```python
from build123d import *

# Parameters (mm, degrees)
BOX015_W                  = 3
BOX015_H                  = 2.5
BOX015_DEPTH              = 1.5
BOX014_W                  = 3
BOX014_H                  = 2.5
BOX014_DEPTH              = 1.5
CYLINDER009_R             = 1.2
CYLINDER009_DEPTH         = 1.54
CYLINDER010_R             = 1.2
CYLINDER010_DEPTH         = 1.54
CYLINDER011_R             = 4.5
CYLINDER011_DEPTH         = 1.54
CYLINDER012_R             = 4.5
CYLINDER012_DEPTH         = 1.54
BOX013_W                  = 18
BOX013_H                  = 16
BOX013_DEPTH              = 1.54
BOX016_W                  = 16.5
BOX016_H                  = 10
BOX016_DEPTH              = 1.54
FUSION014_ROLL_ANGLE      = 180
FUSION014_PLACEMENT_ANGLE = 90.000069


with BuildPart() as cubo015:
    # Box015 → Box015 (new body)
    with BuildSketch(Plane(origin=(12.5, 21.5, 1.54), x_dir=(1, 0, 0), z_dir=(0, 0, 1))):
        with Locations((1.5, 1.25)):
            Rectangle(BOX015_W, BOX015_H)
    extrude(amount=BOX015_DEPTH)


with BuildPart() as cubo014:
    # Box014 → Box014 (new body)
    with BuildSketch(Plane(origin=(3, 21.5, 1.54), x_dir=(1, 0, 0), z_dir=(0, 0, 1))):
        with Locations((1.5, 1.25)):
            Rectangle(BOX014_W, BOX014_H)
    extrude(amount=BOX014_DEPTH)


with BuildPart() as cilindro008:
    # Cylinder009 → Cylinder009 (new body)
    with BuildSketch(Plane(origin=(0, 11.5, 0), x_dir=(1, 0, 0), z_dir=(0, 0, 1))):
        Circle(CYLINDER009_R)
    extrude(amount=CYLINDER009_DEPTH)


with BuildPart() as cilindro009:
    # Cylinder010 → Cylinder010 (new body)
    with BuildSketch(Plane(origin=(18, 11.5, 0), x_dir=(1, 0, 0), z_dir=(0, 0, 1))):
        Circle(CYLINDER010_R)
    extrude(amount=CYLINDER010_DEPTH)


with BuildPart() as cilindro010:
    # Cylinder011 → Cylinder011 (new body)
    with BuildSketch(Plane(origin=(0, 11.5, 0), x_dir=(1, 0, 0), z_dir=(0, 0, 1))):
        Circle(CYLINDER011_R)
    extrude(amount=CYLINDER011_DEPTH)


with BuildPart() as cilindro011:
    # Cylinder012 → Cylinder012 (new body)
    with BuildSketch(Plane(origin=(18, 11.5, 0), x_dir=(1, 0, 0), z_dir=(0, 0, 1))):
        Circle(CYLINDER012_R)
    extrude(amount=CYLINDER012_DEPTH)


with BuildPart() as cubo013:
    # Box013 → Box013 (new body)
    with BuildSketch(Plane.XY):
        with Locations((9, 8)):
            Rectangle(BOX013_W, BOX013_H)
    extrude(amount=BOX013_DEPTH)


with BuildPart() as sensormodel:
    # Box016 → Box016 (new body)
    with BuildSketch(Plane(origin=(1, 16, 0), x_dir=(1, 0, 0), z_dir=(0, 0, 1))):
        with Locations((8.25, 5)):
            Rectangle(BOX016_W, BOX016_H)
    extrude(amount=BOX016_DEPTH)

    # Fusion011: union Cubo013
    add(cubo013.part)

    # Fusion012: union Cilindro011
    add(cilindro011.part)

    # Fusion013: union Cilindro010
    add(cilindro010.part)

    # Cut013: cut Cilindro009
    add(cilindro009.part, mode=Mode.SUBTRACT)

    # Cut014: cut Cilindro008
    add(cilindro008.part, mode=Mode.SUBTRACT)

    # Fusion014: union Cubo015, Cubo014
    add(cubo015.part)
    add(cubo014.part)


with BuildPart() as sensormodel_1:
    # Fusion014 roll: moved
    add(sensormodel.part.rotate(Axis((0, 0, 0), (1, 0, 0)), FUSION014_ROLL_ANGLE))


with BuildPart() as sensormodel_2:
    # Fusion014 placement: moved
    add(sensormodel_1.part.moved(Location((-22.790785, -25.673595, 18.5))).rotate(Axis((-22.790785, -25.673595, 18.5), (0, 0, 1)), FUSION014_PLACEMENT_ANGLE))


solid = sensormodel_2.part
```
Verification items for the finished model (mm, model axes). Round coordinates to 2 decimals unless told otherwise and drop trailing zeros. Order: outer loops, then holes, each group sorted by start corner. A loop starts at its lowest first (then second) coordinate and runs counter-clockwise, first axis right, second up. Notation, with made-up numbers: (12, -13) -> (30, -13) arc R26 ccw to (30, 11) -> close; hole circle Ø4 at (85.5, -19). An arc over 180 degrees is marked (long way). Put each result on its own line as item: value. Start each with the question number.
(1) Section check A-A (z = 16.6). Enter the section's corners in (x, y), then the cut area to 3 significant figures.
(2) Section check D-D (y = -17.5). Enter the section's corners in (x, z), then the cut area to 3 significant figures.
(3) Material ranges on line 1 along X through (y, z) = (-25.75, 17.55); line 2 along Y through (x, z) = (0.5, 16.05); line 3 along Y through (x, z) = (-11.5, 17.85), recorded low to high.
(4) Draft check along X on faces 1 (the face through (0, -12, 15.46)), 2 (the face through (-11.39, -3.175, 17.741)), 3 (the face through (-12.021, -26.626, 17.741)). Enter one of: +X half, -X half, draft (parallel to the pull), parting line (faces both ways), or undercut.
(5) Section check C-C (x = -21). Enter the section's corners in (y, z).
(6) Section check B-B (y = -12). Enter the section's corners in (x, z), then the cut area to 3 significant figures.
(7) Depth check by flat-ended pin: pin 1 Ø1.2 at (x, z) = (0, 16.5) entering from +Y; pin 2 Ø12 at (x, y) = (-17.5, -7) entering from +Z; pin 3 Ø1.7 at (x, z) = (-19.5, 17.5) entering from +Y; pin 4 Ø13 at (x, y) = (-10.5, -14.5) entering from -Z. Enter the tip coordinate at first touch or a pass-through.
Completed:
1. outline: (-1.29, -22.67) -> (1.21, -22.67) -> (1.21, -19.67) -> (-1.29, -19.67) -> close; (-1.29, -13.17) -> (1.21, -13.17) -> (1.21, -10.17) -> (-1.29, -10.17) -> close
1. area: 15.0 mm2
2. outline: (-22.79, 16.96) -> (3.21, 16.96) -> (3.21, 18.5) -> (-22.79, 18.5) -> close
2. area: 40.0 mm2
3. line 1: x = -15.79 to -12.49, -10.09 to -6.79
3. line 2: y = -22.67 to -19.67, -13.17 to -10.17
3. line 3: y = -30.17 to -26.86, -24.49 to -8.86, -6.49 to -3.18
4. face 1: draft
4. face 2: parting line
4. face 3: undercut
5. outline: (-25.67, 16.96) -> (-7.67, 16.96) -> (-7.67, 18.5) -> (-25.67, 18.5) -> close
6. outline: (-22.79, 16.96) -> (-1.29, 16.96) -> (-1.29, 15.46) -> (1.21, 15.46) -> (1.21, 16.96) -> (3.21, 16.96) -> (3.21, 18.5) -> (-22.79, 18.5) -> close
6. area: 43.8 mm2
7. pin 1: stops at y = -8.17
7. pin 2: stops at z = 18.5
7. pin 3: stops at y = -7.67
7. pin 4: stops at z = 16.96
